```python
from build123d import *

# Parameters (mm, degrees)
SKETCH1_W           = 1620
SKETCH1_H           = 1620
SKETCH1_W_2         = 500
SKETCH1_H_2         = 500
BOSS_EXTRUDE1_DEPTH = 300
SKETCH2_W           = 1620
SKETCH2_H           = 1620
SKETCH2_W_2         = 500
SKETCH2_H_2         = 500
BOSS_EXTRUDE2_DEPTH = 3
SKETCH3_W           = 1620
SKETCH3_H           = 1620
SKETCH3_W_2         = 500
SKETCH3_H_2         = 500
BOSS_EXTRUDE3_DEPTH = 3


with BuildPart() as part:
    # Sketch1 → Boss-Extrude1 (new body)
    with BuildSketch(Plane.XY):
        with Locations((-207.337883959, -81.092150171)):
            Rectangle(SKETCH1_W, SKETCH1_H)
        with Locations((-747.337883959, -621.092150171)):
            Rectangle(SKETCH1_W_2, SKETCH1_H_2, mode=Mode.SUBTRACT)
        with Locations((-207.337883959, -621.092150171)):
            Rectangle(SKETCH1_W_2, SKETCH1_H_2, mode=Mode.SUBTRACT)
        with Locations((-747.337883959, -81.092150171)):
            Rectangle(SKETCH1_W_2, SKETCH1_H_2, mode=Mode.SUBTRACT)
        with Locations((332.662116041, -81.092150171)):
            Rectangle(SKETCH1_W_2, SKETCH1_H_2, mode=Mode.SUBTRACT)
        with Locations((-747.337883959, 458.907849829)):
            Rectangle(SKETCH1_W_2, SKETCH1_H_2, mode=Mode.SUBTRACT)
        with Locations((-207.337883959, 458.907849829)):
            Rectangle(SKETCH1_W_2, SKETCH1_H_2, mode=Mode.SUBTRACT)
        with Locations((332.662116041, 458.907849829)):
            Rectangle(SKETCH1_W_2, SKETCH1_H_2, mode=Mode.SUBTRACT)
        with Locations((-207.337883959, -81.092150171)):
            Rectangle(SKETCH1_W_2, SKETCH1_H_2, mode=Mode.SUBTRACT)
        with Locations((332.662116041, -621.092150171)):
            Rectangle(SKETCH1_W_2, SKETCH1_H_2, mode=Mode.SUBTRACT)
    extrude(amount=BOSS_EXTRUDE1_DEPTH)

    # Sketch2 → Boss-Extrude2 (add)
    with BuildSketch(Plane.XY.offset(300)):
        with Locations((-207.337883959, -81.092150171)):
            Rectangle(SKETCH2_W, SKETCH2_H)
        with Locations((332.662116041, 458.907849829)):
            Rectangle(SKETCH2_W_2, SKETCH2_H_2, mode=Mode.SUBTRACT)
        with Locations((-747.337883959, 458.907849829)):
            Rectangle(SKETCH2_W_2, SKETCH2_H_2, mode=Mode.SUBTRACT)
        with Locations((-207.337883959, 458.907849829)):
            Rectangle(SKETCH2_W_2, SKETCH2_H_2, mode=Mode.SUBTRACT)
        with Locations((-747.337883959, -81.092150171)):
            Rectangle(SKETCH2_W_2, SKETCH2_H_2, mode=Mode.SUBTRACT)
        with Locations((-207.337883959, -81.092150171)):
            Rectangle(SKETCH2_W_2, SKETCH2_H_2, mode=Mode.SUBTRACT)
        with Locations((332.662116041, -81.092150171)):
            Rectangle(SKETCH2_W_2, SKETCH2_H_2, mode=Mode.SUBTRACT)
        with Locations((-747.337883959, -621.092150171)):
            Rectangle(SKETCH2_W_2, SKETCH2_H_2, mode=Mode.SUBTRACT)
        with Locations((-207.337883959, -621.092150171)):
            Rectangle(SKETCH2_W_2, SKETCH2_H_2, mode=Mode.SUBTRACT)
        with Locations((332.662116041, -621.092150171)):
            Rectangle(SKETCH2_W_2, SKETCH2_H_2, mode=Mode.SUBTRACT)
    extrude(amount=BOSS_EXTRUDE2_DEPTH)

    # Sketch3 → Boss-Extrude3 (add)
    with BuildSketch(Plane(origin=(0, 0, 0), x_dir=(-1, 0, 0), z_dir=(0, 0, -1))):
        with Locations((207.337883959, -81.092150171)):
            Rectangle(SKETCH3_W, SKETCH3_H)
        with Locations((747.337883959, -621.092150171)):
            Rectangle(SKETCH3_W_2, SKETCH3_H_2, mode=Mode.SUBTRACT)
        with Locations((207.337883959, -621.092150171)):
            Rectangle(SKETCH3_W_2, SKETCH3_H_2, mode=Mode.SUBTRACT)
        with Locations((-332.662116041, -621.092150171)):
            Rectangle(SKETCH3_W_2, SKETCH3_H_2, mode=Mode.SUBTRACT)
        with Locations((207.337883959, -81.092150171)):
            Rectangle(SKETCH3_W_2, SKETCH3_H_2, mode=Mode.SUBTRACT)
        with Locations((-332.662116041, -81.092150171)):
            Rectangle(SKETCH3_W_2, SKETCH3_H_2, mode=Mode.SUBTRACT)
        with Locations((207.337883959, 458.907849829)):
            Rectangle(SKETCH3_W_2, SKETCH3_H_2, mode=Mode.SUBTRACT)
        with Locations((747.337883959, -81.092150171)):
            Rectangle(SKETCH3_W_2, SKETCH3_H_2, mode=Mode.SUBTRACT)
        with Locations((747.337883959, 458.907849829)):
            Rectangle(SKETCH3_W_2, SKETCH3_H_2, mode=Mode.SUBTRACT)
        with Locations((-332.662116041, 458.907849829)):
            Rectangle(SKETCH3_W_2, SKETCH3_H_2, mode=Mode.SUBTRACT)
    extrude(amount=BOSS_EXTRUDE3_DEPTH)


solid = part.part
```
Part model, mm, in its own coordinate system. Give positions to 0.01 mm unless a question says otherwise; leave off trailing zeros. Loops run counter-clockwise (first coordinate to the right, second up) from the corner with the lowest first, then second, coordinate; pieces in that order, holes last. Notation, with made-up numbers: M 65,7 L 95,7 A13 ccw 95,23 Z; hole C 30,7.5 d9. An arc over 180 degrees is marked long. Return JSON: item names as keys, results as strings.
1) Saw through at A-A, the plane y = -85. List the corners of the cut face in (x, z), then the cut area to 3 significant figures.
Calculated:
{"outline": "M -1017.34,-3 L -997.34,-3 L -997.34,303 L -1017.34,303 Z; M -497.34,-3 L -457.34,-3 L -457.34,303 L -497.34,303 Z; M 42.66,-3 L 82.66,-3 L 82.66,303 L 42.66,303 Z; M 582.66,-3 L 602.66,-3 L 602.66,303 L 582.66,303 Z", "area": "36,700 mm2"}
2) Drill centre lines: line 1 (X direction, y = 388, z = 214); line 2 (Y direction, x = -910, z = 190.5). Where is each one in solid material? Low to high.
Calculated:
{"line 1": "x = -1017.34 to -997.34, -497.34 to -457.34, 42.66 to 82.66, 582.66 to 602.66", "line 2": "y = -891.09 to -871.09, -371.09 to -331.09, 168.91 to 208.91, 708.91 to 728.91"}
3) Pull direction Y, two halves, no side cores. Call faces 1 (the face through (-204, -331.092, 152)), 2 (the face through (-457.338, -625, 152)), 3 (the face through (-1017.338, -92, 152)): released by +Y, released by -Y, zero draft, split by the parting line, or undercut.
Calculated:
{"face 1": "undercut", "face 2": "undercut", "face 3": "zero draft"}
4) Saw through at C-C, the plane z = 108. Count the separate pieces of the cut face and the enclosed holes in it, then the cut area to 3 significant figures.
Calculated:
{"separate pieces": "1", "enclosed holes": "9", "area": "374,000 mm2"}
5) Saw through at B-B, the plane x = -594. List the corners of the cut face in (y, z).
Calculated:
{"outline": "M -891.09,-3 L -871.09,-3 L -871.09,303 L -891.09,303 Z; M -371.09,-3 L -331.09,-3 L -331.09,303 L -371.09,303 Z; M 168.91,-3 L 208.91,-3 L 208.91,303 L 168.91,303 Z; M 708.91,-3 L 728.91,-3 L 728.91,303 L 708.91,303 Z"}
